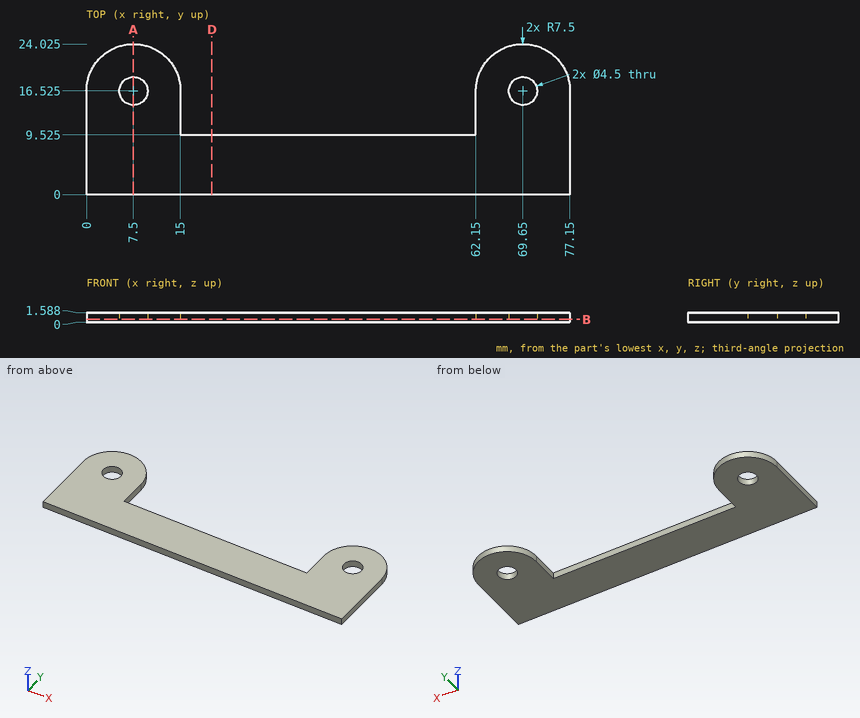
The figure shows three views and two pictorial views of one solid part (mm, origin at its lowest corner). Answer the questions. Give positions to 0.01 mm unless a question says otherwise; leave off trailing zeros. Order: outer loops, then holes, each group sorted by start corner. A loop starts at its lowest first (then second) coordinate and runs counter-clockwise, first axis right, second up. Notation, with made-up numbers: M 67.25,4 L 96.25,4 A21 cw 96.25,20 Z; hole C 41,6.5 d5. An arc over 180 degrees is marked long. Return JSON: item names as keys, results as strings.
Q1. Each of these flat-tipped pins is pushed along its axis until it touches: pin 1 (3.5 mm diameter, centred on x = 7.5, y = 16.525, fed in from -Z); pin 2 (0.5 mm diameter, centred on x = 40.5, z = 0.5, fed in from +Y) (1 decimal). Where does it stop, or does it pass through?
Answer below:
{"pin 1": "passes through", "pin 2": "stops at y = 9.5"}
Q2. Find section B-B, the plane z = 0.5. State how many separate pieces and enclosed holes the cut face has, and give its area (3 significant figures).
Answer below:
{"separate pieces": "1", "enclosed holes": "2", "area": "1,090 mm^2"}
Q3. Find section A-A, the plane x = 7.5. Write down the section's boundary in (y, z) (1 decimal), and give its area (3 significant figures).
Answer below:
{"outline": "M 0,0 L 14.3,0 L 14.3,1.6 L 0,1.6 Z; M 18.8,0 L 24,0 L 24,1.6 L 18.8,1.6 Z", "area": "31.0 mm^2"}
Q4. Find section D-D, the plane x = 20. Write down the section's boundary in (y, z) (1 decimal).
Answer below:
{"outline": "M 0,0 L 9.5,0 L 9.5,1.6 L 0,1.6 Z"}
Q5. Find the intervals of material crossed by line 1 along X through (y, z) = (16.75, 0.5); line 2 along Y through (x, z) = (7.5, 0.9) (1 decimal); line 3 along X through (y, z) = (11, 0.15), in increasing order. Write a range as [from, to].
Answer below:
{"line 1": "x = [0, 5.26], [9.74, 15], [62.15, 67.41], [71.89, 77.15]", "line 2": "y = [0, 14.3], [18.8, 24]", "line 3": "x = [0, 15], [62.15, 77.15]"}
